The figure shows three views and two pictorial views of one solid part (mm, origin at its lowest corner). Answer the questions. Round coordinates to 2 decimals unless told otherwise and drop trailing zeros. Write each loop counter-clockwise with the first axis right and the second up, starting at its lowest first coordinate (ties: lowest second). Pieces come first, ordered by that corner, then holes. Notation, with made-up numbers: (48, 67.25) -> (76, 67.25) arc R17 cw to (76, 97.25) -> close; hole circle Ø7 at (34.5, 25). An arc over 180 degrees is marked (long way). One line per item, written item: value.
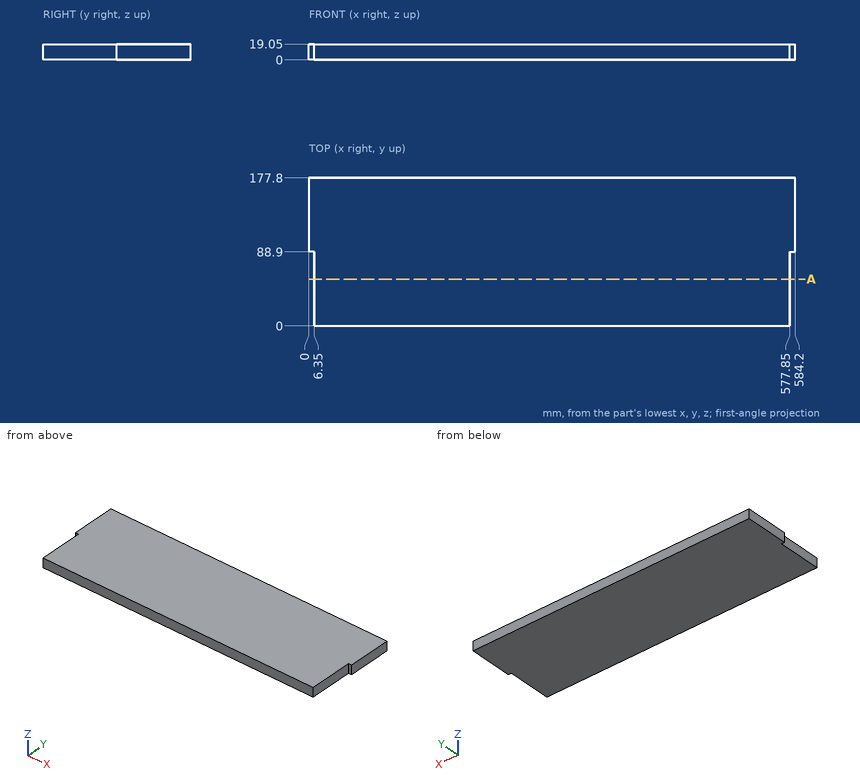
(1) Consider probe 1 along X at (y, z) = (66.5, 11.5). Determine where the line is inside the solid, lowest interval first.
Reported:
probe 1: x = 6.35 to 577.85
(2) Find section A-A on y = 56. Give the vertices of the cut face in (x, z).
Reported:
outline: (6.35, 0) -> (577.85, 0) -> (577.85, 19.05) -> (6.35, 19.05) -> close
(3) Flat-ended cylindrical pins translate along their axes: pin 1 Ø3 at (x, z) = (579.5, 8.5) entering from -Y; pin 2 Ø9.5 at (y, z) = (35, 11.5) entering from -X; pin 3 Ø9.5 at (y, z) = (51, 9.5) entering from +X. Find the tip coordinate at first contact, or state that the pin passes through.
Reported:
pin 1: stops at y = 88.9
pin 2: stops at x = 6.35
pin 3: stops at x = 577.85
